Model file for the job. Use its own axes, mm. Face numbers are marked on the shaded views. A direction names the side the tool comes from. Round coordinates to 2 decimals unless told otherwise and drop trailing zeros. Order: outer loops, then holes, each group sorted by start corner. A loop starts at its lowest first (then second) coordinate and runs counter-clockwise, first axis right, second up. Notation, with made-up numbers: (28.5, 84.25) - (44.5, 84.25) arc R22 cw to (44.5, 119.25) - close; hole circle Ø2 at (15.5, 89.5). An arc over 180 degrees is marked (long way). Put each result on its own line as item: value. Start each with the question number.
Item 1: Probe probe 1 along Y at (x, z) = (-3.75, -3.75); probe 2 along Z at (x, y) = (-2, 2.75); probe 3 along Z at (x, y) = (4.75, 1.5). List the from-to ranges inside material, lowest first.
Item 2: Which spindle directions (+Z, -Z, +X, -X, +Y, -Y) get a long thin tool onto all of the face, cutting with end or side? Do the marked faces 1, 2 and 3. Say none if no direction does.
Item 3: Saw through at A-A on z = 0. List the corners of the cut face in (x, y), plus the area to 3 significant figures.
Item 4: Saw through at D-D on x = -7.75. List the corners of the cut face in (y, z).
Item 5: Saw through at B-B on x = 0. List the corners of the cut face in (y, z), plus the area to 3 significant figures.
Item 6: Pin check, flat tip, straight feed: pin 1 Ø5 at (x, z) = (0.5, -3) entering from -Y. Stop position of the tip, or through.
Item 7: Saw through at C-C on y = 1. List the corners of the cut face in (x, z).
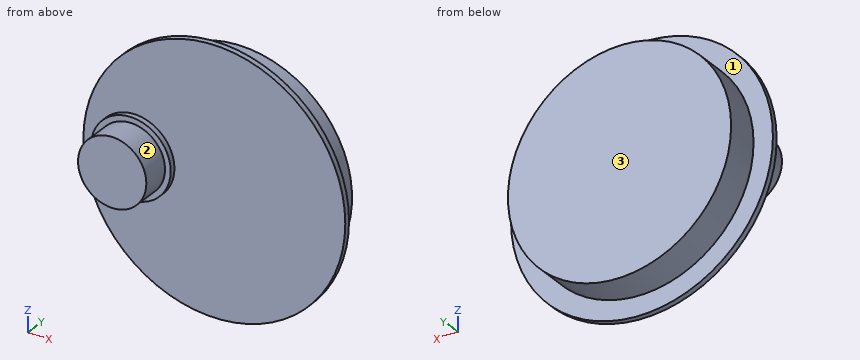
Autodesk Inventor part; units mm, degrees
ref_plane "YZ Plane" through (0, 0, 0) normal (1, 0, 0) x (0, 1, 0)
ref_plane "XZ Plane" through (0, 0, 0) normal (0, 1, 0) x (-1, 0, 0)
ref_plane "XY Plane" through (0, 0, 0) normal (0, 0, 1) x (1, 0, 0)
sketch "スケッチ1" plane through (0, 0, 0) normal (0, 1, 0) x (-1, 0, 0)
  circle A0 centre (0, 0) radius 9.8
  dimension "d0" = 19.6
extrude "押し出し1" add sketch "スケッチ1" along normal blind 3
sketch "スケッチ2" plane through (0, 0, 0) normal (0, -1, 0) x (1, 0, 0)
  circle A0 centre (-7, 0) radius 3
  circle A1 centre (-7, 0) radius 3.5
  circle A2 centre (0, 0) radius 10
  dimension "d3" = 6
  dimension "d6" = 7
  dimension "d12" = 20
extrude "押し出し2" add sketch "スケッチ2" along normal blind 3.5 contours A0
extrude "押し出し3" add sketch "スケッチ2" along normal blind 1 contours A2 A1 | A2 A1 picked at (-3.7315, -0.526) picked at (-10.3053, -0.2541)
sketch "スケッチ3" plane through (0, 0, 0) normal (0, -1, 0) x (1, 0, 0)
  circle A0 centre (0, 0) radius 11.5
  dimension "d9" = 23
extrude "押し出し4" add sketch "スケッチ3" along normal blind 0.5
properties part number "wrist_hone_upper_cover"
Results found:
1. probe 1: y = -0.5 to 3
1. probe 2: z = -9.59 to 9.59
1. probe 3: z = -8.57 to 8.57
2. face 1: +Y
2. face 2: -Y
2. face 3: +Z, -Z, +X, -X, +Y
3. outline: (-11.5, -0.5) - (-10.5, -0.5) - (-10.5, -1) - (-10, -1) - (-10, -3.5) - (-4, -3.5) - (-4, -1) - (-3.5, -1) - (-3.5, -0.5) - (11.5, -0.5) - (11.5, 0) - (9.8, 0) - (9.8, 3) - (-9.8, 3) - (-9.8, 0) - (-11.5, 0) - close
3. area: 88.8 mm²
4. outline: (-3.5, -2.9) - (-1, -2.9) - (-1, -3.42) - (-0.5, -3.42) - (-0.5, -8.5) - (0, -8.5) - (0, -6) - (3, -6) - (3, 6) - (0, 6) - (0, 8.5) - (-0.5, 8.5) - (-0.5, 3.42) - (-1, 3.42) - (-1, 2.9) - (-3.5, 2.9) - close
5. outline: (-0.5, -11.5) - (0, -11.5) - (0, -9.8) - (3, -9.8) - (3, 9.8) - (0, 9.8) - (0, 11.5) - (-0.5, 11.5) - close
5. area: 70.3 mm²
6. pin 1: stops at y = -0.5
7. outline: circle Ø19.6 at (0, 0)
